from build123d import *

# Parameters (mm, degrees)
BOSS_EXTRUDE1_DEPTH     = 54
CUT_EXTRUDE1_DEPTH      = 61.464865831
CUT_EXTRUDE1_DEPTH_BACK = 61.464865831
SKETCH2_R               = 2
SKETCH2_4_R             = 3.1
SKETCH2_4_R_2           = 2
CUT_EXTRUDE2_DEPTH      = 5
CUT_EXTRUDE7_DEPTH      = 64.348243944
CUT_EXTRUDE7_DEPTH_BACK = 64.348243944
FILLET1_R               = 1
FILLET2_R               = 10


with BuildPart() as part:
    # Sketch1 → Boss-Extrude1 (new body)
    with BuildSketch(Plane(origin=(0, 0, 0), x_dir=(0, 0, -1), z_dir=(1, 0, 0))):
        with BuildLine():
            Line((16, 8), (16, 19.627416998))
            Line((16, 19.627416998), (6.627416998, 29))
            Line((6.627416998, 29), (-6.627416998, 29))
            Line((-6.627416998, 29), (-16, 19.627416998))
            Line((-16, 19.627416998), (-16, 8))
            ThreePointArc((-16, 8), (-15.242535625, 7.0298575), (-14.117647059, 7.529411765))
            ThreePointArc((-14.117647059, 7.529411765), (0, 16), (14.117647059, 7.529411765))
            ThreePointArc((14.117647059, 7.529411765), (15.242535625, 7.0298575), (16, 8))
        make_face()
    extrude(amount=BOSS_EXTRUDE1_DEPTH)

    # Sketch2 → Cut-Extrude1 (cut, two sides: drawn at the far end of the back side and taken through both)
    with BuildSketch(Plane(origin=(0, 29, 0), x_dir=(1, 0, 0), z_dir=(0, 1, 0)).offset(-CUT_EXTRUDE1_DEPTH_BACK)):
        with Locations(Location((9, 0, 0), (0, 0, 270))):
            Circle(SKETCH2_R)
        with Locations(Location((21, 0, 0), (0, 0, 270))):
            Circle(SKETCH2_R)
        with Locations(Location((33, 0, 0), (0, 0, 270))):
            Circle(SKETCH2_R)
        with Locations(Location((45, 0, 0), (0, 0, 270))):
            Circle(SKETCH2_R)
    extrude(amount=CUT_EXTRUDE1_DEPTH + CUT_EXTRUDE1_DEPTH_BACK, mode=Mode.SUBTRACT)

    # Sketch2_4 → Cut-Extrude2 (cut)
    # profile 1 of 8: a face of its own
    with BuildSketch(Plane(origin=(0, 29, 0), x_dir=(1, 0, 0), z_dir=(0, 1, 0))):
        with Locations(Location((9, 0, 0), (0, 0, 270))):
            Circle(SKETCH2_4_R)
        with Locations(Location((9, 0, 0), (0, 0, 270))):
            Circle(SKETCH2_4_R_2, mode=Mode.SUBTRACT)
    # profile 2 of 8: a face of its own
    with BuildSketch(Plane(origin=(0, 29, 0), x_dir=(1, 0, 0), z_dir=(0, 1, 0))):
        with Locations(Location((9, 0, 0), (0, 0, 270))):
            Circle(SKETCH2_4_R_2)
    # profile 3 of 8: a face of its own
    with BuildSketch(Plane(origin=(0, 29, 0), x_dir=(1, 0, 0), z_dir=(0, 1, 0))):
        with Locations(Location((21, 0, 0), (0, 0, 270))):
            Circle(SKETCH2_4_R)
        with Locations(Location((21, 0, 0), (0, 0, 270))):
            Circle(SKETCH2_4_R_2, mode=Mode.SUBTRACT)
    # profile 4 of 8: a face of its own
    with BuildSketch(Plane(origin=(0, 29, 0), x_dir=(1, 0, 0), z_dir=(0, 1, 0))):
        with Locations(Location((21, 0, 0), (0, 0, 270))):
            Circle(SKETCH2_4_R_2)
    # profile 5 of 8: a face of its own
    with BuildSketch(Plane(origin=(0, 29, 0), x_dir=(1, 0, 0), z_dir=(0, 1, 0))):
        with Locations(Location((33, 0, 0), (0, 0, 270))):
            Circle(SKETCH2_4_R)
        with Locations(Location((33, 0, 0), (0, 0, 270))):
            Circle(SKETCH2_4_R_2, mode=Mode.SUBTRACT)
    # profile 6 of 8: a face of its own
    with BuildSketch(Plane(origin=(0, 29, 0), x_dir=(1, 0, 0), z_dir=(0, 1, 0))):
        with Locations(Location((33, 0, 0), (0, 0, 270))):
            Circle(SKETCH2_4_R_2)
    # profile 7 of 8: a face of its own
    with BuildSketch(Plane(origin=(0, 29, 0), x_dir=(1, 0, 0), z_dir=(0, 1, 0))):
        with Locations(Location((45, 0, 0), (0, 0, 270))):
            Circle(SKETCH2_4_R)
        with Locations(Location((45, 0, 0), (0, 0, 270))):
            Circle(SKETCH2_4_R_2, mode=Mode.SUBTRACT)
    # profile 8 of 8: a face of its own
    with BuildSketch(Plane(origin=(0, 29, 0), x_dir=(1, 0, 0), z_dir=(0, 1, 0))):
        with Locations(Location((45, 0, 0), (0, 0, 270))):
            Circle(SKETCH2_4_R_2)
    extrude(amount=-CUT_EXTRUDE2_DEPTH, mode=Mode.SUBTRACT)

    # Sketch4 → Cut-Extrude7 (cut, two sides: drawn at the far end of the back side and taken through both)
    with BuildSketch(Plane.ZY.offset(-CUT_EXTRUDE7_DEPTH_BACK)):
        with BuildLine():
            Line((-5, 21), (-5, 15.198684154))
            ThreePointArc((-5, 15.198684154), (0, 16), (5, 15.198684154))
            Line((5, 15.198684154), (5, 21))
            Line((5, 21), (-5, 21))
        make_face()
    extrude(amount=CUT_EXTRUDE7_DEPTH + CUT_EXTRUDE7_DEPTH_BACK, mode=Mode.SUBTRACT)

    # Fillet1
    fillet1_edges = [part.edges().sort_by_distance(p)[0] for p in [
        (27, 15.198684154, -5),
        (27, 21, -5),
        (27, 15.198684154, 5),
        (27, 21, 5),
        (27, 29, -6.627416998),
        (27, 29, 6.627416998),
    ]]
    fillet(fillet1_edges, radius=FILLET1_R)

    # Fillet2
    fillet2_edges = [part.edges().sort_by_distance(p)[0] for p in [
        (27, 19.627416998, -16),
        (27, 19.627416998, 16),
    ]]
    fillet(fillet2_edges, radius=FILLET2_R)


solid = part.part
Input: part model. Units: mm. Frame: model coordinates. A direction names the side the tool comes from. Give positions to 0.01 mm unless a question says otherwise; leave off trailing zeros. Order: outer loops, then holes, each group sorted by start corner. A loop starts at its lowest first (then second) coordinate and runs counter-clockwise, first axis right, second up. Notation, with made-up numbers: (-10, 49) - (44, 49) arc R20 cw to (44, 69) - close; hole circle Ø2 at (-39, 15). An arc over 180 degrees is marked (long way). Answer as a JSON object with one key per item and string values. Group by question number.
Q1. Cut plane A-A, the plane x = 9. Output: boundary loops of the cut face in (y, z).
Q2. First-contact query: pin 1 Ø7 at (x, z) = (9, 0) entering from -Y; pin 2 Ø5 at (x, y) = (23.5, 25.5) entering from -Z; pin 3 Ø6.5 at (x, z) = (33, 0) entering from +Y; pin 4 Ø1.5 at (x, z) = (34.5, -9) entering from -Y. Flat tips, straight axial feed; report the tip coordinate or a pass-through.
Q3. Cut plane C-C, the plane x = 16.5. Output: boundary loops of the cut face in (y, z).
Q4. Mould query, pull axis X, two halves, no side actions, for faces 4 (the face through (11, 22, 0)), 5 (the face through (0, 23, 0)), 6 (the face through (27, 12, -16)). Classes: pulls with the +X half, pulls with the -X half, needs draft (parallel to the pull), parting line crosses it, or undercut.
Q5. Line query: probe 1 along X at (y, z) = (22.7, 0); probe 2 along X at (y, z) = (28, 0); probe 3 along Z at (x, y) = (46, 16). Output: solid intervals per line, ascending.
Q6. Cut plane D-D, the plane z = 0. Count the separate pieces of the cut face and the enclosed holes in it, then the cut area to 3 significant figures.
Q7. Cut plane B-B, the plane y = 9. Output: boundary loops of the cut face in (x, z).
Q8. Set-up query: faces 1 (the face through (11.61, 26.54, 1.67)), 2 (the face through (27, 12, 16)), 3 (the face through (26.622, 20.699, -4.715)). Return all of +Z, -Z, +X, -X, +Y, -Y with unobstructed straight access to the full face (end or side cutting, diameter ignored); none if empty.
Results:
{
 "1": {"outline": "(7.53, -14.12) arc R1 ccw to (8, -16) - (15.49, -16) arc R10 ccw to (22.56, -13.07) - (28.71, -6.92) arc R1 ccw to (29, -6.21) - (29, -3.1) - (24, -3.1) - (24, -2) - (21, -2) - (21, -4) arc R1 cw to (20, -5) - (15.91, -5) arc R1 ccw to (14.97, -5.65) arc R16 cw to start; (7.53, 14.12) arc R16 cw to (14.97, 5.65) arc R1 ccw to (15.91, 5) - (20, 5) arc R1 cw to (21, 4) - (21, 2) - (24, 2) - (24, 3.1) - (29, 3.1) - (29, 6.21) arc R1 ccw to (28.71, 6.92) - (22.56, 13.07) arc R10 ccw to (15.49, 16) - (8, 16) arc R1 ccw to start"},
 "2": {"pin 1": "y = 21", "pin 2": "z = -12.63", "pin 3": "y = 29", "pin 4": "y = 12.69"},
 "3": {"outline": "(7.53, -14.12) arc R1 ccw to (8, -16) - (15.49, -16) arc R10 ccw to (22.56, -13.07) - (28.71, -6.92) arc R1 ccw to (29, -6.21) - (29, 6.21) arc R1 ccw to (28.71, 6.92) - (22.56, 13.07) arc R10 ccw to (15.49, 16) - (8, 16) arc R1 ccw to (7.53, 14.12) arc R16 cw to (14.97, 5.65) arc R1 ccw to (15.91, 5) - (20, 5) arc R1 cw to (21, 4) - (21, -4) arc R1 cw to (20, -5) - (15.91, -5) arc R1 ccw to (14.97, -5.65) arc R16 cw to start"},
 "4": {"face 4": "undercut", "face 5": "pulls with the -X half", "face 6": "needs draft"},
 "5": {"probe 1": "0 to 7, 11 to 19, 23 to 31, 35 to 43, 47 to 54", "probe 2": "0 to 5.9, 12.1 to 17.9, 24.1 to 29.9, 36.1 to 41.9, 48.1 to 54", "probe 3": "-15.99 to -5, 5 to 15.99"},
 "6": {"separate pieces": "5", "enclosed holes": "0", "area": "260 mm^2"},
 "7": {"outline": "(0, -16) - (54, -16) - (54, -13.23) - (0, -13.23) - close; (0, 13.23) - (54, 13.23) - (54, 16) - (0, 16) - close"},
 "8": {"face 1": "+Y", "face 2": "+Z, +X, -X, +Y, -Y", "face 3": "+X, -X, -Y"}
}
